from build123d import *

# Parameters (mm, degrees)
SKETCH1_R                = 12.5
SKETCH1_R_2              = 4.25
BOSS_EXTRUDE1_DEPTH      = 2.5
BOSS_EXTRUDE2_START      = 5
BOSS_EXTRUDE2_DEPTH      = 5
BOSS_EXTRUDE3_DEPTH      = 50
BOSS_EXTRUDE3_DEPTH_BACK = 50
SKETCH3_R                = 10
CUT_EXTRUDE1_START       = -40
SKETCH4_R                = 4.25
CUT_EXTRUDE1_DEPTH       = 40


with BuildPart() as part:
    # Sketch1 → Boss-Extrude1 (new body)
    with BuildSketch(Plane.XY):
        Circle(SKETCH1_R)
        Circle(SKETCH1_R_2, mode=Mode.SUBTRACT)
    extrude(amount=BOSS_EXTRUDE1_DEPTH)

    # Sketch2 → Boss-Extrude2 (add)
    with BuildSketch(Plane(origin=(0, 0, 0), x_dir=(-1, 0, 0), z_dir=(0, 0, -1)).offset(BOSS_EXTRUDE2_START)):
        with BuildLine():
            ThreePointArc((-6.106396375, 10.906966733), (10.50822507, 6.769579446), (7.406819033, -10.069212075))
            add(Edge.make_bspline(
                [(7.406819033, -10.069212075), (-7.979907505, -21.387545439), (-26.855730435, -52.646283336), (-9.439793984, -88.354039493), (6.611094261, -102.497105047)],
                knots=[0, 0, 0, 0, 0.455821989, 1, 1, 1, 1], degree=3))
            ThreePointArc((6.611094261, -102.497105047), (7.323414251, -116.809376161), (-7.00278738, -117.138695182))
            add(Edge.make_bspline(
                [(-6.106396375, 10.906966733), (-20.621715475, 2.78039093), (-57.030134585, -32.014511607), (-40.003016754, -84.766730291), (-7.00278738, -117.138695182)],
                knots=[0, 0, 0, 0, 0.30202419, 1, 1, 1, 1], degree=3))
        make_face()
    extrude(amount=-BOSS_EXTRUDE2_DEPTH)

    # Sketch3 → Boss-Extrude3 (add, two sides: drawn at the far end of the back side and taken through both)
    with BuildSketch(Plane.XY.offset(-BOSS_EXTRUDE3_DEPTH_BACK)):
        with Locations((0, -110)):
            Circle(SKETCH3_R)
    extrude(amount=BOSS_EXTRUDE3_DEPTH + BOSS_EXTRUDE3_DEPTH_BACK)

    # Sketch4 → Cut-Extrude1 (cut)
    with BuildSketch(Plane.XY.offset(CUT_EXTRUDE1_START)):
        Circle(SKETCH4_R)
    extrude(amount=CUT_EXTRUDE1_DEPTH, mode=Mode.SUBTRACT)


solid = part.part
The model under review builds one solid part; all positions refer to its coordinate system, in mm. A direction names the side the tool comes from. Round coordinates to 2 decimals unless told otherwise and drop trailing zeros. Order: outer loops, then holes, each group sorted by start corner. A loop starts at its lowest first (then second) coordinate and runs counter-clockwise, first axis right, second up. Notation, with made-up numbers: (-3.75, 34) -> (23.25, 34) arc R21 ccw to (23.25, 69) -> close; hole circle Ø10 at (-8.5, 78). An arc over 180 degrees is marked (long way). Write item = value, one per line. Start each with the question number.
Item 1: Consider section B-B on x = 2.5. Count the separate pieces of the cut face and the enclosed holes in it, plus the area to 3 significant figures.
Item 2: For faces 1 (the face through (0, -110, 50)), 2 (the face through (0, -5, 2.5)), 3 (the face through (-8, -116, -1)), list the 3-axis set-ups (+Z, -Z, +X, -X, +Y, -Y) from which the entire face can be reached by the end or side of a thin tool; tool diameter is ignored.
Item 3: Clearance check with flat-ended pins moving along their axes: pin 1 Ø12.5 at (x, y) = (0, 3.5) entering from +Z; pin 2 Ø3 at (y, z) = (-81, -8) entering from -X; pin 3 Ø3 at (x, z) = (-2.5, -40) entering from +Y; pin 4 Ø12 at (y, z) = (-11, 7.5) entering from -X. State where each tip first meets the part, or that it passes through.
Item 4: Consider section A-A on z = -23. Write out the cut boundary in (x, y), plus the area to 3 significant figures.
Item 5: Mouldability with a two-part tool opening along Y and no side actions: class faces 4 (the face through (2.285, 3.584, -1.303)), 5 (the face through (22, -37, -5)) as released by +Y, released by -Y, zero draft, split by the parting line, or undercut.
Item 6: For line 1 along Y through (x, z) = (0, 0.5); line 2 along Y through (x, z) = (0, -2); line 3 along X through (y, z) = (0, 0.75), list the stretches that pass through material, from the lowest coordinate up.
Conclusion:
q1.separate_pieces = 3
q1.enclosed_holes = 0
q1.area = 2,140 mm2
q2.face_1 = +Z, +X, -X, +Y, -Y
q2.face_2 = +Z, +X, -X, +Y
q2.face_3 = none
q3.pin_1 = 2.5
q3.pin_2 = through
q3.pin_3 = -100.05
q3.pin_4 = -9.86
q4.outline = circle Ø20 at (0, -110)
q4.area = 314 mm2
q5.face_4 = undercut
q5.face_5 = zero draft
q6.line_1 = -120 to -100, -12.5 to -4.25, 4.25 to 12.5
q6.line_2 = -120 to -95.97, -16.23 to -4.25, 4.25 to 12.5
q6.line_3 = -12.5 to -4.25, 4.25 to 12.5
